The model under review builds one solid part; all positions refer to its coordinate system, in mm. Face numbers are marked on the shaded views. A direction names the side the tool comes from. Round coordinates to 2 decimals unless told otherwise and drop trailing zeros. Order: outer loops, then holes, each group sorted by start corner. A loop starts at its lowest first (then second) coordinate and runs counter-clockwise, first axis right, second up.
Autodesk Inventor part; units mm, degrees
ref_plane "YZ Plane" through (0, 0, 0) normal (1, 0, 0) x (0, 1, 0)
ref_plane "XZ Plane" through (0, 0, 0) normal (0, 1, 0) x (-1, 0, 0)
ref_plane "XY Plane" through (0, 0, 0) normal (0, 0, 1) x (1, 0, 0)
sketch "Эскиз1" plane through (0, 0, 0) normal (0, 0, 1) x (1, 0, 0)
  circle A0 centre (0, 0) radius 5
  dimension "d0" = 10
extrude "Выдавливание1" add sketch "Эскиз1" along normal blind 6
sketch "Эскиз2" plane through (0, 0, 6) normal (0, 0, 1) x (1, 0, 0)
  circle A0 centre (0, 0) radius 5
  line L0 (0, 5.6569) -> (5.6569, 0)
  line L1 (5.6569, 0) -> (0, -5.6569)
  line L2 (0, -5.6569) -> (-5.6569, 0)
  line L3 (-5.6569, 0) -> (0, 5.6569)
  dimension "d3" = 8
extrude "Выдавливание2" cut sketch "Эскиз2" against normal blind 6 contours A0 L1 L2 L3 L0 | A0 L0 L1 | A0 L3 L0 | L1 L2 A0 | A0 L2 L3 keep common part
sketch "Эскиз3" plane through (0, 0, 6) normal (0, 0, 1) x (1, 0, 0)
  line L0 (-0.7071, -4.9497) -> (-4.9497, -0.7071)
  arc A0 (-0.7071, -4.9497) -> (0.7071, -4.9497) centre (0, 0) ccw
  line L1 (4.9497, -0.7071) -> (0.7071, -4.9497)
  arc A1 (4.9497, -0.7071) -> (4.9497, 0.7071) centre (0, 0) ccw
  line L2 (0.7071, 4.9497) -> (4.9497, 0.7071)
  arc A2 (0.7071, 4.9497) -> (-0.7071, 4.9497) centre (0, 0) ccw
  line L3 (-4.9497, 0.7071) -> (-0.7071, 4.9497)
  arc A3 (-4.9497, 0.7071) -> (-4.9497, -0.7071) centre (0, 0) ccw
  circle A4 centre (0, 0) radius 8
  dimension "d6" = 16
extrude "Выдавливание3" add sketch "Эскиз3" along normal blind 3
sketch "Эскиз4" plane through (0, 0, 9) normal (0, 0, 1) x (1, 0, 0)
  arc A0 (-4.9497, 0.7071) -> (-4.9497, -0.7071) centre (0, 0) ccw
  line L0 (-4.9497, 0.7071) -> (-0.7071, 4.9497)
  arc A1 (0.7071, 4.9497) -> (-0.7071, 4.9497) centre (0, 0) ccw
  line L1 (0.7071, 4.9497) -> (4.9497, 0.7071)
  arc A2 (4.9497, -0.7071) -> (4.9497, 0.7071) centre (0, 0) ccw
  line L2 (4.9497, -0.7071) -> (0.7071, -4.9497)
  arc A3 (-0.7071, -4.9497) -> (0.7071, -4.9497) centre (0, 0) ccw
  line L3 (-0.7071, -4.9497) -> (-4.9497, -0.7071)
extrude "Выдавливание4" add sketch "Эскиз4" against normal blind 3
sketch "Эскиз5" plane through (0, 0, 9) normal (0, 0, 1) x (1, 0, 0)
  circle A0 centre (0, 0) radius 8
  circle A1 centre (0, 0) radius 5
  dimension "d11" = 10
extrude "Выдавливание5" add sketch "Эскиз5" along normal blind 39 contours A1
sketch "Эскиз6" plane through (0, 0, 48) normal (0, 0, 1) x (1, 0, 0)
  circle A0 centre (0, 0) radius 5
sketch "Эскиз7" plane through (0, 0, 48) normal (0, 0, 1) x (1, 0, 0)
  circle A0 centre (0, 0) radius 5
properties part number "Поз12 Стержень"
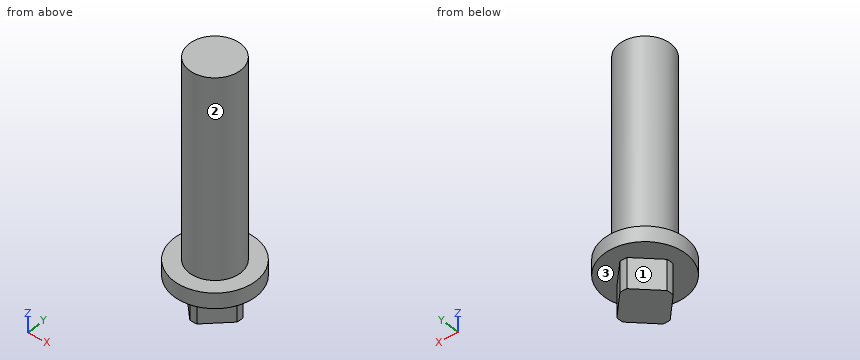
(1) Clearance check with flat-ended pins moving along their axes: P1, Ø8, axis at x = 6, y = 6, coming from the -Z side; P2, Ø2, axis at x = -6, y = 1.5, coming from the +Z side; P3, Ø6, axis at x = -4.5, z = 22.5, coming from the -Y side; P4, Ø1, axis at y = -6, z = 34.5, coming from the -X side. State where each tip first meets the part, or that it passes through.
(2) We need section C-C (z = 16). Give the boundary of the cut face in (x, y).
(3) Tool access review of the marked faces 1, 2 and 3: name each direction out of +Z, -Z, +X, -X, +Y, -Y from which nothing blocks a thin tool from reaching the whole face with its end or side.
(4) To check wall thickness, follow L1, parallel to Z at x = -4, y = 2.5; L2, parallel to Z at x = 7.25, y = 0.5; L3, parallel to Y at x = 0.25, z = 20.5. State the ranges of each line that lie inside material, in increasing order.
(5) We need section A-A (y = 0). Give the boundary of the cut face in (x, z).
(6) We need section D-D (z = 8). Give the boundary of the cut face in (x, y).
Verdict:
1. P1: stops at z = 6
1. P2: stops at z = 9
1. P3: stops at y = -4.77
1. P4: passes through
2. outline: circle Ø10 at (0, 0)
3. face 1: -Z, -X, +Y
3. face 2: +Z
3. face 3: -Z
4. L1: z = 6 to 48
4. L2: z = 6 to 9
4. L3: y = -4.99 to 4.99
5. outline: (-8, 6) - (-5, 6) - (-5, 0) - (5, 0) - (5, 6) - (8, 6) - (8, 9) - (5, 9) - (5, 48) - (-5, 48) - (-5, 9) - (-8, 9) - close
6. outline: circle Ø16 at (0, 0)
